```python
from build123d import *

# Parameters (mm, degrees)
SALIENTE_EXTRUIR1_DEPTH = 10
CROQUIS3_W              = 15
CROQUIS3_H              = 25
CORTAR_EXTRUIR1_DEPTH   = 20


with BuildPart() as part:
    # Croquis2 → Saliente-Extruir1 (new body, symmetric)
    with BuildSketch(Plane.XY):
        Polygon((-10, 15), (-50, -15), (-10, -15), (10, -15), (50, -15), (10, 15), align=None)
    extrude(amount=SALIENTE_EXTRUIR1_DEPTH, both=True)

    # Croquis3 → Cortar-Extruir1 (cut)
    with BuildSketch(Plane.XY.offset(10)):
        with Locations((0, 2.5)):
            Rectangle(CROQUIS3_W, CROQUIS3_H)
    extrude(amount=-CORTAR_EXTRUIR1_DEPTH, mode=Mode.SUBTRACT)


solid = part.part
```
Part model, mm, in its own coordinate system. A direction names the side the tool comes from. Give positions to 0.01 mm unless a question says otherwise; leave off trailing zeros. Write each loop counter-clockwise with the first axis right and the second up, starting at its lowest first coordinate (ties: lowest second). Pieces come first, ordered by that corner, then holes. Notation, with made-up numbers: (58.5, 47.5) -> (84.5, 47.5) arc R18 ccw to (84.5, 74.5) -> close; hole circle Ø6 at (58.5, 74.5). An arc over 180 degrees is marked (long way). Put each result on its own line as item: value. Start each with the question number.
Item 1: Wall check: L1, parallel to Y at x = 3, z = 1.25; L2, parallel to X at y = -4, z = -3.5; L3, parallel to X at y = 9, z = -7.5. Give the ranges that are in metal, low to high. Write a range as [from, to].
Item 2: Cut at A-A (y = -8.25). List the corners of the cut face in (x, z), then the cut area to 3 significant figures.
Item 3: Which spindle directions (+Z, -Z, +X, -X, +Y, -Y) get a long thin tool onto all of the face, cutting with end or side? Do faces 5 (the face through (-30, 0, 0)), 6 (the face through (-7.5, 2, 0)). Say none if no direction does.
Item 4: Cut at C-C (x = -31). List the corners of the cut face in (y, z).
Item 5: Pull direction X, two halves, no side cores. Call faces 1 (the face through (0, -10, 0)), 2 (the face through (-9, 15, 0)), 3 (the face through (7.5, 2, 0)), 4 (the face through (30, 0, 0)): pulls with the +X half, pulls with the -X half, needs draft (parallel to the pull), parting line crosses it, or undercut.
Item 6: Cut at D-D (y = 3.5). List the corners of the cut face in (x, z), then the cut area to 3 significant figures.
Item 7: Pin check, flat tips, straight feed: pin 1 Ø1.5 at (y, z) = (6.5, -7) entering from -X; pin 2 Ø3 at (x, z) = (3, -0.5) entering from +Y; pin 3 Ø4 at (x, z) = (32.5, -4.5) entering from +Y (3 decimals). Stop position of each tip, or through.
Item 8: Cut at B-B (z = -5.5). List the corners of the cut face in (x, y).
Answer list:
1. L1: y = [-15, -10]
1. L2: x = [-35.33, -7.5], [7.5, 35.33]
1. L3: x = [-18, -7.5], [7.5, 18]
2. outline: (-41, -10) -> (-7.5, -10) -> (-7.5, 10) -> (-41, 10) -> close; (7.5, -10) -> (41, -10) -> (41, 10) -> (7.5, 10) -> close
2. area: 1,340 mm2
3. face 5: +Z, -Z, -X, +Y
3. face 6: +Z, -Z, +Y
4. outline: (-15, -10) -> (-0.75, -10) -> (-0.75, 10) -> (-15, 10) -> close
5. face 1: undercut
5. face 2: needs draft
5. face 3: undercut
5. face 4: pulls with the +X half
6. outline: (-25.33, -10) -> (-7.5, -10) -> (-7.5, 10) -> (-25.33, 10) -> close; (7.5, -10) -> (25.33, -10) -> (25.33, 10) -> (7.5, 10) -> close
6. area: 713 mm2
7. pin 1: stops at x = -22.33
7. pin 2: stops at y = -10
7. pin 3: stops at y = -0.375
8. outline: (-50, -15) -> (50, -15) -> (10, 15) -> (7.5, 15) -> (7.5, -10) -> (-7.5, -10) -> (-7.5, 15) -> (-10, 15) -> close
